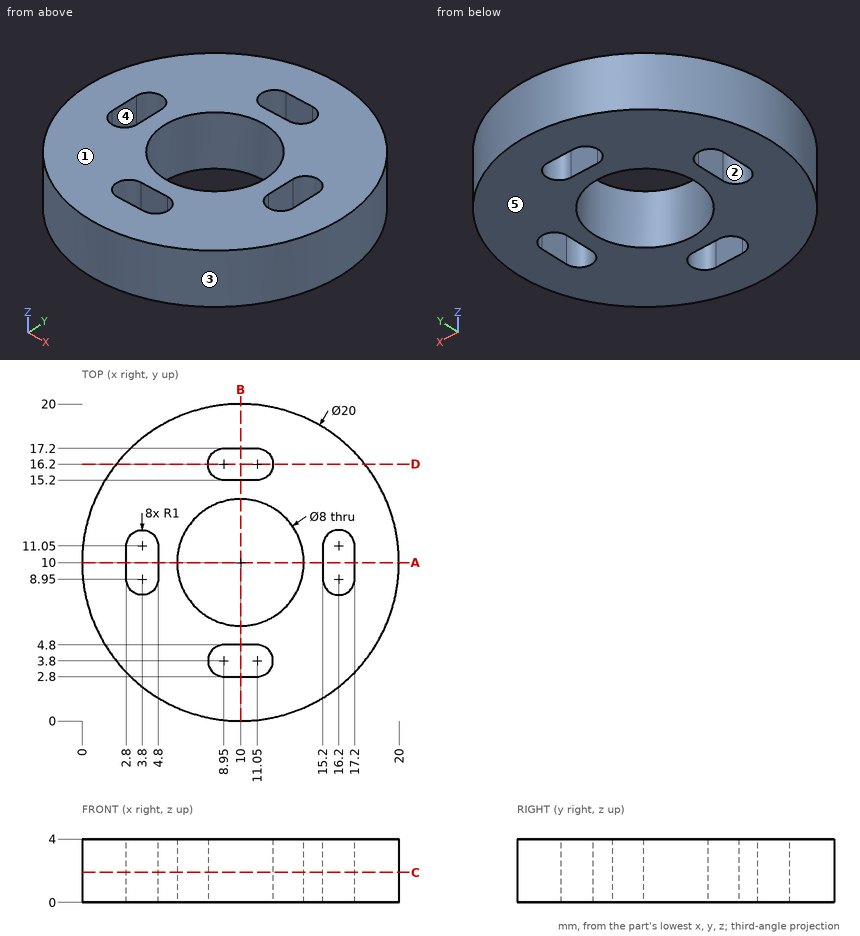
Drawing for the job (mm, zero at the part's lowest x, y, z). A direction names the side the tool comes from. Round coordinates to 2 decimals unless told otherwise and drop trailing zeros. Write each loop counter-clockwise with the first axis right and the second up, starting at its lowest first coordinate (ties: lowest second). Pieces come first, ordered by that corner, then holes. Notation, with made-up numbers: (71.5, 28) - (123.5, 28) arc R28 ccw to (123.5, 53) - close; hole circle Ø1 at (10, 35.25). An arc over 180 degrees is marked (long way). Write item = value, one per line. Start each with the question number.
Q1. Band-saw the part on D-D (y = 16.2). Give the cut face in (x, z).
Q2. Band-saw the part on A-A (y = 10). Give the cut face in (x, z).
Q3. Which spindle directions (+Z, -Z, +X, -X, +Y, -Y) get a long thin tool onto all of the face, cutting with end or side? Do the marked faces 1 and 2. Say none if no direction does.
Q4. Band-saw the part on C-C (z = 1.9). Give the cut face in (x, y).
Q5. Probe L1, parallel to Y at x = 10, z = 1.2; L2, parallel to X at y = 9, z = 2.15; L3, parallel to X at y = 11.75, z = 0.35. List the from-to ranges inside material, lowest first. Write a range as from..to.
Q6. Drop a flat-ended pin along its axis: pin 1 (0.6 mm diameter, centred on y = 10.5, z = 1, fed in from +X). Give the stop position or say it passes through.
Q7. Mould opens along X. For the marked faces 3, 4 and 5 say: pulls with the +X half, pulls with the -X half, needs draft (parallel to the pull), parting line crosses it, or undercut.
Answers below:
q1.outline = (2.15, 0) - (7.95, 0) - (7.95, 4) - (2.15, 4) - close; (12.05, 0) - (17.85, 0) - (17.85, 4) - (12.05, 4) - close
q2.outline = (0, 0) - (2.8, 0) - (2.8, 4) - (0, 4) - close; (4.8, 0) - (6, 0) - (6, 4) - (4.8, 4) - close; (14, 0) - (15.2, 0) - (15.2, 4) - (14, 4) - close; (17.2, 0) - (20, 0) - (20, 4) - (17.2, 4) - close
q3.face_1 = +Z, +X, -X, +Y, -Y
q3.face_2 = +Z, -Z
q4.outline = circle Ø20 at (10, 10); hole (2.8, 8.95) arc R1 ccw to (4.8, 8.95) - (4.8, 11.05) arc R1 ccw to (2.8, 11.05) - close; hole circle Ø8 at (10, 10); hole (8.95, 2.8) - (11.05, 2.8) arc R1 ccw to (11.05, 4.8) - (8.95, 4.8) arc R1 ccw to start; hole (8.95, 15.2) - (11.05, 15.2) arc R1 ccw to (11.05, 17.2) - (8.95, 17.2) arc R1 ccw to start; hole (15.2, 8.95) arc R1 ccw to (17.2, 8.95) - (17.2, 11.05) arc R1 ccw to (15.2, 11.05) - close
q5.L1 = 0..2.8, 4.8..6, 14..15.2, 17.2..20
q5.L2 = 0.05..2.8, 4.8..6.13, 13.87..15.2, 17.2..19.95
q5.L3 = 0.15..3.09, 4.51..6.4, 13.6..15.49, 16.91..19.85
q6.pin_1 = 20
q7.face_3 = parting line crosses it
q7.face_4 = undercut
q7.face_5 = needs draft
